Input: part model. Units: mm. Frame: model coordinates. A direction names the side the tool comes from. Round coordinates to 2 decimals unless told otherwise and drop trailing zeros. Loops run counter-clockwise (first coordinate to the right, second up) from the corner with the lowest first, then second, coordinate; pieces in that order, holes last. Notation, with made-up numbers: M 11,28 L 27,28 A31 cw 27,63 Z; hole C 15,49 d3. An arc over 180 degrees is marked long. Use one line per item in the form item = value. Start each with the question number.
Q1. Section query C-C, the plane z = -0.25. Output: boundary loops of the cut face in (x, y) (3 decimals).
Q2. Ray query, line 1 along Z through (x, y) = (0, -1.9); line 2 along Z through (x, y) = (5.75, 0.3) (3 decimals); line 3 along X through (y, z) = (0.7, 0.5) (3 decimals). Return the intervals inside material, ascending.
Q3. Section query D-D, the plane x = -3.25. Output: boundary loops of the cut face in (y, z) (3 decimals).
Q4. First-contact query: P1, Ø2, axis at x = 0, z = -0.5, coming from the -Y side; P2, Ø2, axis at y = -2, z = -2, coming from the -X side (3 decimals); P3, Ø1.5, axis at y = -2.5, z = 1.5, coming from the -X side. Flat tips, straight axial feed; report the tip coordinate or a pass-through.
Q5. Section query B-B, the plane x = 0. Output: boundary loops of the cut face in (y, z) (3 decimals).
Q6. Section query A-A, the plane y = 0.5. Output: boundary loops of the cut face in (x, z) (3 decimals).
Q7. Access query for faces 1 (the cylindrical face through (-0.5, -2.1, -2.4)), 2 (the flat face through (0, 1.2, 0)), 3 (the flat face through (6.475, 1, 0)). Directions: +Z, -Z, +X, -X, +Y, -Y. A direction counts if a zero-diameter tool reaches every point of the face in a straight line with its end or side. Return the directions, or none.
Q8. Mould query, pull axis Z, two halves, no side actions, for faces 4 (the flat face through (0, 0, 3.925)), 5 (the flat face through (-2, -1.2, 2)), 6 (the cylindrical face through (1.5, 0.59, 0.07)). Classes: pulls with the +Z half, pulls with the -Z half, needs draft (parallel to the pull), parting line crosses it, or undercut.
```python
from build123d import *

# Parameters (mm, degrees)
F0_W     = 15.85
F0_H     = 7.85
F1_DEPTH = 1.2
F2_R     = 2.45
F2_R_2   = 2
F3_DEPTH = 1.8
F4_W     = 15.85
F4_H     = 7.85
F4_W_2   = 12.95
F4_H_2   = 4.95
F4_R     = 1.5
F5_DEPTH = 1.2


with BuildPart() as f1:
    # F0 (on Front) → F1 (new body)
    with BuildSketch(Plane.XZ):
        Rectangle(F0_W, F0_H)
    extrude(amount=F1_DEPTH)

    # F2 (on face) → F3 (join)
    with BuildSketch(Plane.XZ.offset(1.2)):
        Circle(F2_R)
        Circle(F2_R_2, mode=Mode.SUBTRACT)
    extrude(amount=F3_DEPTH)

    # F4 (on face) → F5 (join)
    with BuildSketch(Plane(origin=(0, 0, 0), x_dir=(-1, 0, 0), z_dir=(0, 1, 0))):
        Rectangle(F4_W, F4_H)
        Rectangle(F4_W_2, F4_H_2, mode=Mode.SUBTRACT)
        Circle(F4_R)
    extrude(amount=F5_DEPTH)


solid = f1.part
```
Results found:
q1.outline = M -7.925,-1.2 L -2.437,-1.2 L -2.437,-3 L -1.984,-3 L -1.984,-1.2 L 1.984,-1.2 L 1.984,-3 L 2.437,-3 L 2.437,-1.2 L 7.925,-1.2 L 7.925,1.2 L 6.475,1.2 L 6.475,0 L 1.479,0 L 1.479,1.2 L -1.479,1.2 L -1.479,0 L -6.475,0 L -6.475,1.2 L -7.925,1.2 Z
q2.line_1 = -2.45 to -2, 2 to 2.45
q2.line_2 = -3.925 to -2.475, 2.475 to 3.925
q2.line_3 = -7.925 to -6.475, -1.414 to 1.414, 6.475 to 7.925
q3.outline = M -1.2,-3.925 L 1.2,-3.925 L 1.2,-2.475 L 0,-2.475 L 0,2.475 L 1.2,2.475 L 1.2,3.925 L -1.2,3.925 Z
q4.P1 = -1.2
q4.P2 = -7.925
q4.P3 = -2.33
q5.outline = M -3,-2.45 L -1.2,-2.45 L -1.2,-3.925 L 1.2,-3.925 L 1.2,-2.475 L 0,-2.475 L 0,-1.5 L 1.2,-1.5 L 1.2,1.5 L 0,1.5 L 0,2.475 L 1.2,2.475 L 1.2,3.925 L -1.2,3.925 L -1.2,2.45 L -3,2.45 L -3,2 L -1.2,2 L -1.2,-2 L -3,-2 Z
q6.outline = M -7.925,-3.925 L 7.925,-3.925 L 7.925,3.925 L -7.925,3.925 Z; C 0,0 d3; hole M -6.475,-2.475 L 6.475,-2.475 L 6.475,2.475 L -6.475,2.475 Z
q7.face_1 = -Y
q7.face_2 = +Z, -Z, +X, -X, +Y
q7.face_3 = +Y
q8.face_4 = pulls with the +Z half
q8.face_5 = needs draft
q8.face_6 = undercut
